```python
from build123d import *

# Parameters (mm, degrees)
SKETCH1_W                                       = 89.09
SKETCH1_H                                       = 62.42
SKETCH1_W_2                                     = 85.09
SKETCH1_H_2                                     = 58.42
BOSS_EXTRUDE1_DEPTH                             = 2
SKETCH1_3_W                                     = 89.09
SKETCH1_3_H                                     = 62.42
SKETCH1_3_W_2                                   = 85.09
SKETCH1_3_H_2                                   = 58.42
BOSS_EXTRUDE2_DEPTH                             = 10
CSK_FOR_M2_FLAT_HEAD_MACHINE_SCREW1_D           = 1.8
CSK_FOR_M2_FLAT_HEAD_MACHINE_SCREW1_DEPTH       = 9.906
CSK_FOR_M2_FLAT_HEAD_MACHINE_SCREW1_CSINK_D     = 4.4
CSK_FOR_M2_FLAT_HEAD_MACHINE_SCREW1_CSINK_ANGLE = 90
CSK_FOR_M2_FLAT_HEAD_MACHINE_SCREW1_TIP         = 0.540774557
SKETCH7_W                                       = 41.935160688
SKETCH7_H                                       = 41.279429724
CUT_EXTRUDE1_DEPTH                              = 2.54


with BuildPart() as part:
    # Sketch1 → Boss-Extrude1 (new body)
    # profile 1 of 2: a face of its own
    with BuildSketch(Plane(origin=(0, 0, 0), x_dir=(1, 0, 0), z_dir=(0, 1, 0))):
        Rectangle(SKETCH1_W, SKETCH1_H)
        Rectangle(SKETCH1_W_2, SKETCH1_H_2, mode=Mode.SUBTRACT)
    # profile 2 of 2: a face of its own
    with BuildSketch(Plane(origin=(0, 0, 0), x_dir=(1, 0, 0), z_dir=(0, 1, 0))):
        Rectangle(SKETCH1_W_2, SKETCH1_H_2)
    extrude(amount=-BOSS_EXTRUDE1_DEPTH)

    # Sketch1_3 → Boss-Extrude2 (add)
    with BuildSketch(Plane(origin=(0, 0, 0), x_dir=(1, 0, 0), z_dir=(0, 1, 0))):
        Rectangle(SKETCH1_3_W, SKETCH1_3_H)
        Rectangle(SKETCH1_3_W_2, SKETCH1_3_H_2, mode=Mode.SUBTRACT)
    extrude(amount=BOSS_EXTRUDE2_DEPTH)

    # CSK for M2 Flat Head Machine Screw1
    with Locations(Plane(origin=(0, 0, 0), x_dir=(1, 0, 0), z_dir=(0, 1, 0))):
        with Locations((37.5, 7.335501447), (-37.5, 7.335501447), (-37.5, -7.664498553), (37.5, -7.664498553)):
            CounterSinkHole(CSK_FOR_M2_FLAT_HEAD_MACHINE_SCREW1_D / 2, CSK_FOR_M2_FLAT_HEAD_MACHINE_SCREW1_CSINK_D / 2, depth=CSK_FOR_M2_FLAT_HEAD_MACHINE_SCREW1_DEPTH, counter_sink_angle=CSK_FOR_M2_FLAT_HEAD_MACHINE_SCREW1_CSINK_ANGLE)
            with Locations((0, 0, -(CSK_FOR_M2_FLAT_HEAD_MACHINE_SCREW1_DEPTH + CSK_FOR_M2_FLAT_HEAD_MACHINE_SCREW1_TIP / 2))):  # 118° drill point
                Cone(0, CSK_FOR_M2_FLAT_HEAD_MACHINE_SCREW1_D / 2, CSK_FOR_M2_FLAT_HEAD_MACHINE_SCREW1_TIP, mode=Mode.SUBTRACT)

    # Sketch7 → Cut-Extrude1 (cut)
    with BuildSketch(Plane(origin=(0, 0, 0), x_dir=(1, 0, 0), z_dir=(0, 1, 0))):
        Rectangle(SKETCH7_W, SKETCH7_H)
    extrude(amount=-CUT_EXTRUDE1_DEPTH, mode=Mode.SUBTRACT)


solid = part.part
```
For this review, take the finished solid that the model builds, in its own axes (mm). A direction names the side the tool comes from. Coordinates: 2 decimals unless noted, no trailing zeros. Write each loop counter-clockwise with the first axis right and the second up, starting at its lowest first coordinate (ties: lowest second). Pieces come first, ordered by that corner, then holes. Notation, with made-up numbers: (61, 75) - (102, 75) arc R25 cw to (102, 96) - close; hole circle Ø11 at (78.5, 32). An arc over 180 degrees is marked (long way). Answer in a Markdown table with one row per item. Add a question column.
Q1. We need section D-D, the plane y = 1. State the section outline as (x, z) points (3 decimals).
Q2. Tool access review of faces 4 (the flat face through (0, -1, -20.64)), 5 (the flat face through (-44.545, 4, 0)), 6 (the flat face through (-1, 5, -29.21)): name each direction out of +Z, -Z, +X, -X, +Y, -Y from which nothing blocks a thin tool from reaching the whole face with its end or side.
Q3. We need section B-B, the plane x = -16. State the section outline as (y, z) points, and give its area (3 significant figures).
Q4. For probe 1 along X at (y, z) = (8, -24.5) (3 decimals); probe 2 along Z at (x, y) = (37.5, -1.65); probe 3 along Z at (x, y) = (-30.5, 5.5), list the stretches that pass through material, from the lowest coordinate up.
Q5. We need section A-A, the plane z = 11. State the section outline as (x, y) points (3 decimals).
Q6. For P1, Ø1.5, axis at x = 27, z = -11, coming from the +Y side; P2, Ø2, axis at x = 37.5, z = 7.66, coming from the -Y side, all flat-tipped, find the tip position at first contact; note any pin that passes through.
Q7. Draft analysis for pull direction Z (two halves, no side actions). For faces 1 (the flat face through (-1, 4, 31.21)), 2 (the flat face through (-20.968, -1, 0)), 3 (the flat face through (44.545, 4, 0)), state which applies: +Z half, -Z half, draft (parallel to the pull), parting line (faces both ways), or undercut.
Q8. We need section C-C, the plane x = -37.5. State the section outline as (y, z) points.
Answer list:
| question | item | result |
|---|---|---|
| 1 | outline | (-44.545, -31.21) - (44.545, -31.21) - (44.545, 31.21) - (-44.545, 31.21) - close; hole (-42.545, -29.21) - (42.545, -29.21) - (42.545, 29.21) - (-42.545, 29.21) - close |
| 2 | face 4 | +Y, -Y |
| 2 | face 5 | +Z, -Z, -X, +Y, -Y |
| 2 | face 6 | +Y |
| 3 | outline | (-2, -31.21) - (10, -31.21) - (10, -29.21) - (0, -29.21) - (0, -20.64) - (-2, -20.64) - close; (-2, 20.64) - (0, 20.64) - (0, 29.21) - (10, 29.21) - (10, 31.21) - (-2, 31.21) - close |
| 3 | area | 82.3 mm2 |
| 4 | probe 1 | x = -44.545 to -42.545, 42.545 to 44.545 |
| 4 | probe 2 | z = -31.21 to -8.24, -6.44 to 6.76, 8.56 to 31.21 |
| 4 | probe 3 | z = -31.21 to -29.21, 29.21 to 31.21 |
| 5 | outline | (-44.545, -2) - (-20.968, -2) - (-20.968, 0) - (-42.545, 0) - (-42.545, 10) - (-44.545, 10) - close; (20.968, -2) - (44.545, -2) - (44.545, 10) - (42.545, 10) - (42.545, 0) - (20.968, 0) - close |
| 6 | P1 | stops at y = 0 |
| 6 | P2 | stops at y = -2 |
| 7 | face 1 | +Z half |
| 7 | face 2 | undercut |
| 7 | face 3 | draft |
| 8 | outline | (-2, -31.21) - (10, -31.21) - (10, -29.21) - (0, -29.21) - (0, -9.54) - (-1.3, -8.24) - (-2, -8.24) - close; (-2, -6.44) - (-1.3, -6.44) - (0, -5.14) - (0, 5.46) - (-1.3, 6.76) - (-2, 6.76) - close; (-2, 8.56) - (-1.3, 8.56) - (0, 9.86) - (0, 29.21) - (10, 29.21) - (10, 31.21) - (-2, 31.21) - close |
